```python
from build123d import *

# Parameters (mm, degrees)
BOSS_EXTRUDE1_DEPTH = 3
CUT_EXTRUDE1_DEPTH  = 270.507073191
FILLET1_R           = 2.5
FILLET3_R           = 2.5


with BuildPart() as part:
    # Sketch11 → Boss-Extrude1 (new body)
    with BuildSketch(Plane(origin=(0, 0, 0), x_dir=(1, 0, 0), z_dir=(0, 1, 0))):
        Polygon((250.25, 100), (0, 100), (0, 0), (237.75, 0), align=None)
    extrude(amount=BOSS_EXTRUDE1_DEPTH)

    # Sketch12 → Cut-Extrude1 (cut, through all)
    with BuildSketch(Plane(origin=(0, 3, 0), x_dir=(1, 0, 0), z_dir=(0, 1, 0))):
        with BuildLine():
            Line((14.85, 38.85), (227.15, 38.85))
            ThreePointArc((227.15, 38.85), (232, 34), (227.15, 29.15))
            Line((227.15, 29.15), (14.85, 29.15))
            ThreePointArc((14.85, 29.15), (10, 34), (14.85, 38.85))
        make_face()
        with BuildLine():
            Line((14.85, 86.85), (233.15, 86.85))
            ThreePointArc((233.15, 86.85), (238, 82), (233.15, 77.15))
            Line((233.15, 77.15), (14.85, 77.15))
            ThreePointArc((14.85, 77.15), (10, 82), (14.85, 86.85))
        make_face()
        with BuildLine():
            Line((14.85, 70.85), (231.15, 70.85))
            ThreePointArc((231.15, 70.85), (236, 66), (231.15, 61.15))
            Line((231.15, 61.15), (14.85, 61.15))
            ThreePointArc((14.85, 61.15), (10, 66), (14.85, 70.85))
        make_face()
        with BuildLine():
            Line((14.85, 13.15), (225.15, 13.15))
            ThreePointArc((225.15, 13.15), (230, 18), (225.15, 22.85))
            Line((225.15, 22.85), (14.85, 22.85))
            ThreePointArc((14.85, 22.85), (10, 18), (14.85, 13.15))
        make_face()
        with BuildLine():
            Line((14.85, 54.85), (229.15, 54.85))
            ThreePointArc((229.15, 54.85), (234, 50), (229.15, 45.15))
            Line((229.15, 45.15), (14.85, 45.15))
            ThreePointArc((14.85, 45.15), (10, 50), (14.85, 54.85))
        make_face()
    extrude(amount=-CUT_EXTRUDE1_DEPTH, mode=Mode.SUBTRACT)

    # Fillet1
    fillet1_edges = [part.edges().sort_by_distance(p)[0] for p in [
        (10, 3, -50),
        (122, 3, -45.15),
        (234, 3, -50),
        (122, 3, -54.85),
        (10, 3, -18),
        (120, 3, -13.15),
        (230, 3, -18),
        (120, 3, -22.85),
        (10, 3, -66),
        (123, 3, -61.15),
        (236, 3, -66),
        (123, 3, -70.85),
        (10, 3, -82),
        (124, 3, -77.15),
        (238, 3, -82),
        (124, 3, -86.85),
        (10, 3, -34),
        (121, 3, -29.15),
        (232, 3, -34),
        (121, 3, -38.85),
    ]]
    fillet(fillet1_edges, radius=FILLET1_R)

    # Fillet3
    fillet3_edges = [part.edges().sort_by_distance(p)[0] for p in [
        (237.75, 1.5, 0),
        (0, 1.5, 0),
        (0, 1.5, -100),
        (250.25, 1.5, -100),
    ]]
    fillet(fillet3_edges, radius=FILLET3_R)


solid = part.part
```
Part model, mm, in its own coordinate system. A direction names the side the tool comes from. Give positions to 0.01 mm unless a question says otherwise; leave off trailing zeros. Order: outer loops, then holes, each group sorted by start corner. A loop starts at its lowest first (then second) coordinate and runs counter-clockwise, first axis right, second up. Notation, with made-up numbers: M 86.5,-27 L 139.5,-27 A28 ccw 139.5,-8 Z; hole C 87,84.25 d6. An arc over 180 degrees is marked long. Use a Markdown table: item, result. Add a question column.
(1) 3-axis set-ups, long thin cutter, end or side, ignore diameter. For faces 1 (the face through (123, 0, -40)), 2 (the face through (238, 0.3, -82.1)): which of +Z, -Z, +X, -X, +Y, -Y reach the whole face in a straight line?
(2) Mould opens along X. For faces 3 (the face through (106, 3, -58)), 4 (the face through (10, 0.3, -81.9)), 5 (the face through (243.878, 1.479, -49.025)) say: +X half, -X half, draft (parallel to the pull), parting line (faces both ways), or undercut.
(3) Saw through at C-C, the plane y = 1.5. Give the cut face in (x, z), and give its area (3 significant figures).
(4) Saw through at A-A, the plane z = -82. Give the cut face in (x, y), and give its area (3 significant figures).
(5) Probe line 1 along Z through (x, y) = (83, 0.6); line 2 along Z through (x, y) = (91.5, 1.25); line 3 along X through (y, z) = (1.35, -51.5). List the from-to ranges inside material, lowest first. Write a range as [from, to].
(6) Saw through at B-B, the plane x = 81. Give the number of separate pieces and of enclosed holes in the cut face, and give its area (3 significant figures).
Answer key:
| question | item | result |
|---|---|---|
| 1 | face 1 | +Z, -Z, +X, -X, -Y |
| 1 | face 2 | +Y, -Y |
| 2 | face 3 | draft |
| 2 | face 4 | undercut |
| 2 | face 5 | +X half |
| 3 | outline | M 0,-97.5 A2.5 ccw 2.5,-100 L 247.42,-100 A2.5 ccw 249.9,-97.19 L 238.02,-2.19 A2.5 ccw 235.54,0 L 2.5,0 A2.5 ccw 0,-2.5 Z; hole M 14.85,-87.06 L 233.15,-87.06 A5.06 ccw 233.15,-76.94 L 14.85,-76.94 A5.06 ccw Z; hole M 14.85,-71.06 L 231.15,-71.06 A5.06 ccw 231.15,-60.94 L 14.85,-60.94 A5.06 ccw Z; hole M 14.85,-55.06 L 229.15,-55.06 A5.06 ccw 229.15,-44.94 L 14.85,-44.94 A5.06 ccw Z; hole M 14.85,-39.06 L 227.15,-39.06 A5.06 ccw 227.15,-28.94 L 14.85,-28.94 A5.06 ccw Z; hole M 14.85,-23.06 L 225.15,-23.06 A5.06 ccw 225.15,-12.94 L 14.85,-12.94 A5.06 ccw Z |
| 3 | area | 13,200 mm^2 |
| 4 | outline | M 0,0 L 10,0 L 10,0.5 A2.5 ccw 7.5,3 L 0,3 Z; M 238,0 L 248,0 L 248,3 L 240.5,3 A2.5 ccw 238,0.5 Z |
| 4 | area | 57.3 mm^2 |
| 5 | line 1 | [-100, -86.85], [-77.15, -70.85], [-61.15, -54.85], [-45.15, -38.85], [-29.15, -22.85], [-13.15, 0] |
| 5 | line 2 | [-100, -86.97], [-77.03, -70.97], [-61.03, -54.97], [-45.03, -38.97], [-29.03, -22.97], [-13.03, 0] |
| 5 | line 3 | [0, 10.08], [233.92, 244.19] |
| 6 | separate pieces | 6 |
| 6 | enclosed holes | 0 |
| 6 | area | 141 mm^2 |
